Can you work these out from the drawing? Everything is in mm from the part's minimum corner. Coordinates: 2 decimals unless noted, no trailing zeros. Write each loop counter-clockwise with the first axis right and the second up, starting at its lowest first coordinate (ties: lowest second). Pieces come first, ordered by that corner, then holes. Notation, with made-up numbers: (-35.5, -35) -> (-8.5, -35) arc R10 cw to (-8.5, -17) -> close; hole circle Ø9 at (27.25, 72.5). An arc over 180 degrees is marked (long way). Use a Markdown table: item, result. Add a question column.
Item 1: Will this pin go through, and if not, where does the flat tip stop? pin 1 Ø8 at (x, z) = (22, 8) entering from -Y.
Item 2: Imagine slicing it at A-A, the plane x = 36.5. Write out the boundary of the cut face in (y, z).
Item 3: Imagine slicing it at B-B, the plane z = 2.5. Write out the boundary of the cut face in (x, y), and give its area (3 significant figures).
Item 4: If I drill on line 1 along Z through (x, y) = (36.5, 0.4); line 2 along X through (y, z) = (1.1, 2.5); line 3 along X through (y, z) = (1.4, 33), over which ranges is the centre line in solid material (lowest first)? Write a range as from..to.
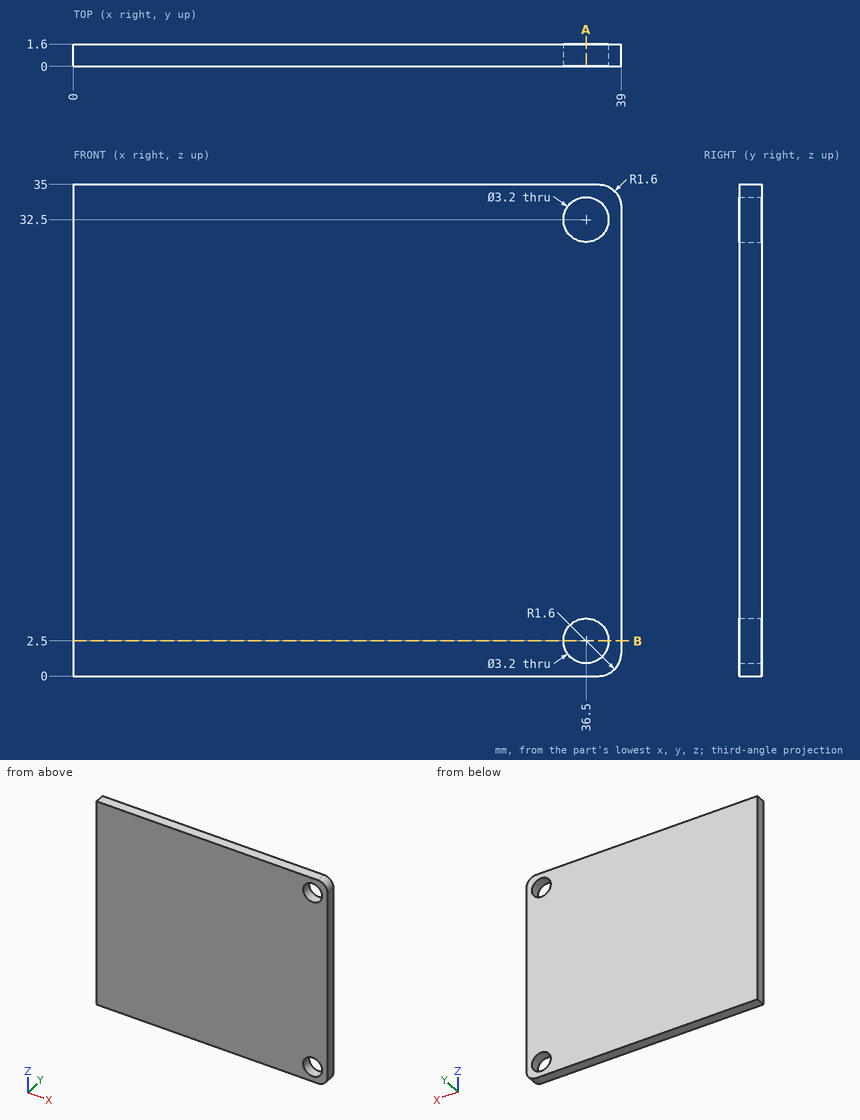
Ans:
| question | item | result |
|---|---|---|
| 1 | pin 1 | stops at y = 0 |
| 2 | outline | (0, 0) -> (1.6, 0) -> (1.6, 0.9) -> (0, 0.9) -> close; (0, 4.1) -> (1.6, 4.1) -> (1.6, 30.9) -> (0, 30.9) -> close; (0, 34.1) -> (1.6, 34.1) -> (1.6, 35) -> (0, 35) -> close |
| 3 | outline | (0, 0) -> (34.9, 0) -> (34.9, 1.6) -> (0, 1.6) -> close; (38.1, 0) -> (39, 0) -> (39, 1.6) -> (38.1, 1.6) -> close |
| 3 | area | 57.3 mm^2 |
| 4 | line 1 | z = 0..0.9, 4.1..30.9, 34.1..35 |
| 4 | line 2 | x = 0..34.9, 38.1..39 |
| 4 | line 3 | x = 0..34.98, 38.02..39 |
